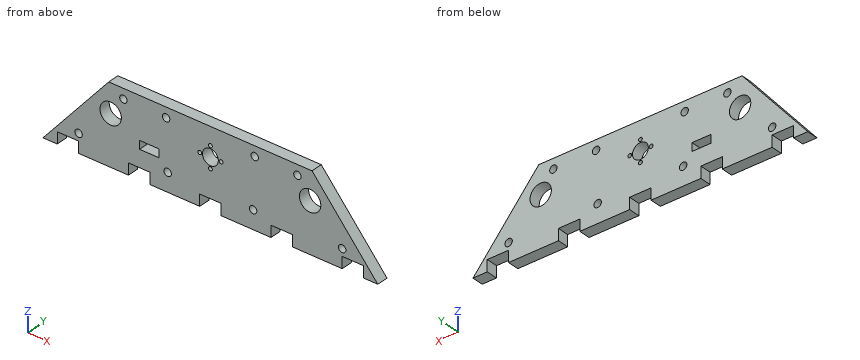
from build123d import *

# Parameters (mm, degrees)
IZIM1_R                              = 2.6821485
IZIM1_R_2                            = 2.780383132
IZIM1_R_3                            = 7.5
IZIM1_R_4                            = 5.187481638
IZIM1_W                              = 13.5
IZIM1_H                              = 5.75
IZIM1_R_5                            = 3.602615137
IZIM1_R_6                            = 4.041767392
Y_KSEKLIK_EKSTR_ZYON1_DEPTH          = 8
M5_HELISARMAL_I_IN_Z_VANA_MATKAB_2_D = 5.2
IZIM13_R                             = 5.55
IZIM13_R_2                           = 1.35
KES_EKSTR_ZYON5_DEPTH                = 10
IZIM14_W                             = 15
IZIM14_H                             = 8
KES_EKSTR_ZYON6_DEPTH                = 8


with BuildPart() as part:
    # Çizim1 → Yükseklik-Ekstrüzyon1 (new body)
    # profile 1 of 9: a face of its own
    with BuildSketch(Plane(origin=(0, 0, 0), x_dir=(1, 0, 0), z_dir=(0, 1, 0))):
        Polygon((-109.77435772, 54.233807267), (-63.623878006, -0.766192733), (7.740916272, -0.766192733), (79.105710549, -0.766192733), (125.256190264, 54.233807267), (7.740916272, 54.233807267), align=None)
        with Locations((-53.338342967, 6.233807267)):
            Circle(IZIM1_R, mode=Mode.SUBTRACT)
        with Locations((-23.338342967, 6.233807267)):
            Circle(IZIM1_R_2, mode=Mode.SUBTRACT)
        with Locations(Location((-62.259083728, 19.233807267, 0), (0, 0, 270))):
            Circle(IZIM1_R_3, mode=Mode.SUBTRACT)
        with Locations((38.820175511, 6.233807267)):
            Circle(IZIM1_R_2, mode=Mode.SUBTRACT)
        with Locations((68.820175511, 6.233807267)):
            Circle(IZIM1_R, mode=Mode.SUBTRACT)
        with Locations(Location((7.740916272, 19.233807267, 0), (0, 0, 270))):
            Circle(IZIM1_R_4, mode=Mode.SUBTRACT)
        with Locations(Location((77.740916272, 19.233807267, 0), (0, 0, 270))):
            Circle(IZIM1_R_3, mode=Mode.SUBTRACT)
        with Locations((-35.200733135, 31.358807267)):
            Rectangle(IZIM1_W, IZIM1_H, mode=Mode.SUBTRACT)
        with Locations((-84.77435772, 41.233807267)):
            Circle(IZIM1_R_5, mode=Mode.SUBTRACT)
        with Locations((-22.259083728, 41.233807267)):
            Circle(IZIM1_R_6, mode=Mode.SUBTRACT)
        with Locations((37.740916272, 41.233807267)):
            Circle(IZIM1_R_6, mode=Mode.SUBTRACT)
        with Locations((100.256190264, 41.233807267)):
            Circle(IZIM1_R_5, mode=Mode.SUBTRACT)
    # profile 2 of 9: a face of its own
    with BuildSketch(Plane(origin=(0, 0, 0), x_dir=(1, 0, 0), z_dir=(0, 1, 0))):
        with Locations((-84.77435772, 41.233807267)):
            Circle(IZIM1_R_5)
    # profile 3 of 9: a face of its own
    with BuildSketch(Plane(origin=(0, 0, 0), x_dir=(1, 0, 0), z_dir=(0, 1, 0))):
        with Locations((-22.259083728, 41.233807267)):
            Circle(IZIM1_R_6)
    # profile 4 of 9: a face of its own
    with BuildSketch(Plane(origin=(0, 0, 0), x_dir=(1, 0, 0), z_dir=(0, 1, 0))):
        with Locations((37.740916272, 41.233807267)):
            Circle(IZIM1_R_6)
    # profile 5 of 9: a face of its own
    with BuildSketch(Plane(origin=(0, 0, 0), x_dir=(1, 0, 0), z_dir=(0, 1, 0))):
        with Locations((100.256190264, 41.233807267)):
            Circle(IZIM1_R_5)
    # profile 6 of 9: a face of its own
    with BuildSketch(Plane(origin=(0, 0, 0), x_dir=(1, 0, 0), z_dir=(0, 1, 0))):
        with Locations((68.820175511, 6.233807267)):
            Circle(IZIM1_R)
    # profile 7 of 9: a face of its own
    with BuildSketch(Plane(origin=(0, 0, 0), x_dir=(1, 0, 0), z_dir=(0, 1, 0))):
        with Locations((38.820175511, 6.233807267)):
            Circle(IZIM1_R_2)
    # profile 8 of 9: a face of its own
    with BuildSketch(Plane(origin=(0, 0, 0), x_dir=(1, 0, 0), z_dir=(0, 1, 0))):
        with Locations((-53.338342967, 6.233807267)):
            Circle(IZIM1_R)
    # profile 9 of 9: a face of its own
    with BuildSketch(Plane(origin=(0, 0, 0), x_dir=(1, 0, 0), z_dir=(0, 1, 0))):
        with Locations((-23.338342967, 6.233807267)):
            Circle(IZIM1_R_2)
    extrude(amount=Y_KSEKLIK_EKSTR_ZYON1_DEPTH)

    # M5 Helisarmal için Zıvana matkabı2 (through all)
    with Locations(Plane(origin=(0, 0, 0), x_dir=(-1, 0, 0), z_dir=(0, -1, 0))):
        with Locations((-68.820175511, 6.233807267), (-38.820175511, 6.233807267), (-37.740916272, 41.233807267), (-100.256190264, 41.233807267), (22.259083728, 41.233807267), (23.338342967, 6.233807267), (53.338342967, 6.233807267), (84.77435772, 41.233807267)):
            Hole(M5_HELISARMAL_I_IN_Z_VANA_MATKAB_2_D / 2)

    # Çizim13 → Kes-Ekstrüzyon5 (cut)
    with BuildSketch(Plane.XZ):
        with Locations(Location((7.740916272, -19.233807267, 0), (0, 0, 270))):
            Circle(IZIM13_R)
        with Locations(Location((15.240916272, -19.233807267, 0), (0, 0, 270))):
            Circle(IZIM13_R_2)
        with Locations(Location((7.740916272, -26.733807267, 0), (0, 0, 270))):
            Circle(IZIM13_R_2)
        with Locations(Location((0.240916272, -19.233807267, 0), (0, 0, 270))):
            Circle(IZIM13_R_2)
        with Locations(Location((7.740916272, -11.733807267, 0), (0, 0, 270))):
            Circle(IZIM13_R_2)
    extrude(amount=-KES_EKSTR_ZYON5_DEPTH, mode=Mode.SUBTRACT)

    # Çizim14 → Kes-Ekstrüzyon6 (cut)
    with BuildSketch(Plane(origin=(0, 0, -54.233807267), x_dir=(-1, 0, 0), z_dir=(0, 0, -1))):
        with Locations((-107.756190264, 4)):
            Rectangle(IZIM14_W, IZIM14_H)
        with Locations((-57.756190264, 4)):
            Rectangle(IZIM14_W, IZIM14_H)
        with Locations((-7.756190264, 4)):
            Rectangle(IZIM14_W, IZIM14_H)
        with Locations((42.243809736, 4)):
            Rectangle(IZIM14_W, IZIM14_H)
        with Locations((92.243809736, 4)):
            Rectangle(IZIM14_W, IZIM14_H)
    extrude(amount=-KES_EKSTR_ZYON6_DEPTH, mode=Mode.SUBTRACT)


solid = part.part
Part model, mm, in its own coordinate system. Round coordinates to 2 decimals unless told otherwise and drop trailing zeros. Loops run counter-clockwise (first coordinate to the right, second up) from the corner with the lowest first, then second, coordinate; pieces in that order, holes last. Notation, with made-up numbers: (76, 35.5) - (80, 35.5) arc R26 ccw to (80, 56.5) - close; hole circle Ø7 at (-23, -24.75). An arc over 180 degrees is marked (long way). Answer as a JSON object with one key per item and string values.
Item 1: Band-saw the part on A-A on x = -59.5. List the corners of the cut face in (y, z).
Output:
{"outline": "(0, -54.23) - (8, -54.23) - (8, -26.21) - (0, -26.21) - close; (0, -12.26) - (8, -12.26) - (8, 0.77) - (0, 0.77) - close"}
Item 2: Wall check: L1, parallel to X at y = 5.5, z = -15; L2, parallel to X at y = 5.5, z = -5.5; L3, parallel to Z at x = -24.5, y = 4. Give the ranges that are in metal, low to high.
Output:
{"L1": "-76.85 to -68.45, -56.07 to 4.15, 11.33 to 71.55, 83.93 to 92.34", "L2": "-68.88 to -55.83, -50.84 to -25.83, -20.84 to 36.33, 41.31 to 66.33, 71.31 to 84.36", "L3": "-54.23 to -42.55, -39.92 to -8.56, -3.91 to 0.77"}
Item 3: Band-saw the part on B-B on y = 6.75. State how many separate pieces and enclosed holes the cut face has, plus the area to 3 significant figures.
Output:
{"separate pieces": "1", "enclosed holes": "16", "area": "9,070 mm2"}
Item 4: Pin check, flat tips, straight feed: pin 1 (4 mm diameter, centred on y = 7, z = -7, fed in from -X); pin 2 (2.5 mm diameter, centred on y = 4, z = -52, fed in from +X); pin 3 (3 mm diameter, centred on y = 4, z = -20, fed in from -X). Stop position of each tip, or through.
Output:
{"pin 1": "x = -71.82", "pin 2": "x = 124.43", "pin 3": "x = -82.31"}
